Verification items for this drawing (mm, ordinates from the low corner). A direction names the side the tool comes from. Coordinates: 2 decimals unless noted, no trailing zeros. Loops run counter-clockwise (first coordinate to the right, second up) from the corner with the lowest first, then second, coordinate; pieces in that order, holes last. Notation, with made-up numbers: (36.25, -26.75) -> (65.25, -26.75) arc R30 ccw to (65.25, -4.75) -> close; hole circle Ø8 at (70.5, 51). An arc over 180 degrees is marked (long way). Write item = value, one per line.
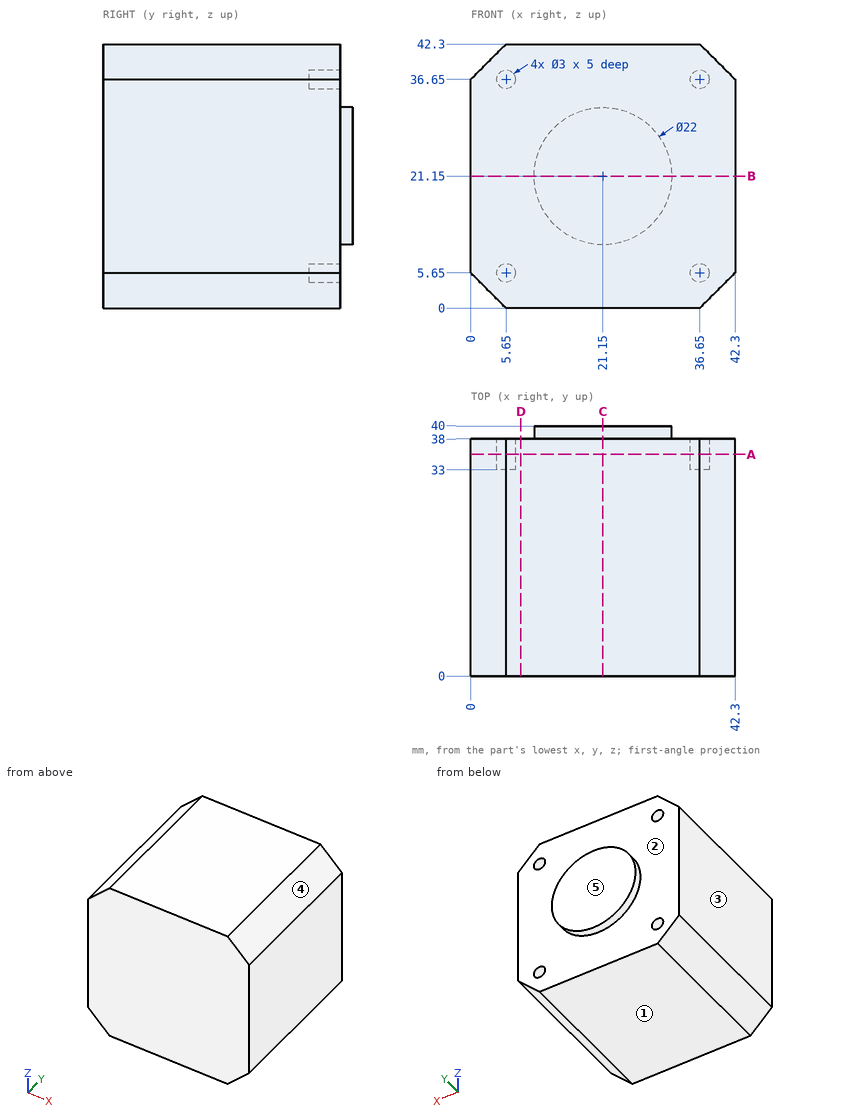
1) Sectioned sample at B-B, the plane z = 21.15. Record the cut outline in (x, y).
Ans:
outline = (0, 0) -> (42.3, 0) -> (42.3, 38) -> (32.15, 38) -> (32.15, 40) -> (10.15, 40) -> (10.15, 38) -> (0, 38) -> close
2) Tool access check on the marked faces 1 and 2. Record the directions out of +Z, -Z, +X, -X, +Y, -Y that give a thin tool (end or side, any length) a straight path to the whole face; none if there is none.
Ans:
face_1 = -Z, +X, -X, +Y, -Y
face_2 = +Y
3) Release check for a two-part mould opening along X. For the marked faces 3, 4 and 5 record: pulls with the +X half, pulls with the -X half, needs draft (parallel to the pull), parting line crosses it, or undercut.
Ans:
face_3 = pulls with the -X half
face_4 = pulls with the +X half
face_5 = needs draft
4) Sectioned sample at D-D, the plane x = 8. Record the cut outline in (y, z).
Ans:
outline = (0, 0) -> (38, 0) -> (38, 42.3) -> (0, 42.3) -> close
5) Material ranges on line 1 (Z direction, x = 5.65, y = 35.3); line 2 (X direction, y = 35, z = 5), recorded low to high.
Ans:
line_1 = 0 to 4.15, 7.15 to 35.15, 38.15 to 42.3
line_2 = 0.65 to 4.3, 7 to 35.3, 38 to 41.65
6) Depth check by flat-ended pin: pin 1 Ø21 at (x, z) = (13, 30.5) entering from +Y; pin 2 Ø2.5 at (x, z) = (36, 36) entering from +Y; pin 3 Ø0.9 at (x, z) = (36, 5) entering from +Y. Enter the tip coordinate at first touch or a pass-through.
Ans:
pin_1 = 40
pin_2 = 38
pin_3 = 33
7) Sectioned sample at A-A, the plane y = 35.5. Record the cut outline in (x, z).
Ans:
outline = (0, 5.65) -> (5.65, 0) -> (36.65, 0) -> (42.3, 5.65) -> (42.3, 36.65) -> (36.65, 42.3) -> (5.65, 42.3) -> (0, 36.65) -> close; hole circle Ø3 at (5.65, 5.65); hole circle Ø3 at (5.65, 36.65); hole circle Ø3 at (36.65, 5.65); hole circle Ø3 at (36.65, 36.65)
8) Sectioned sample at C-C, the plane x = 21.15. Record the cut outline in (y, z).
Ans:
outline = (0, 0) -> (38, 0) -> (38, 10.15) -> (40, 10.15) -> (40, 32.15) -> (38, 32.15) -> (38, 42.3) -> (0, 42.3) -> close
